from build123d import *

# Parameters (mm, degrees)
SKETCH1_R           = 1.651
BOSS_EXTRUDE1_DEPTH = 3.175
FILLET2_R           = 2.54


with BuildPart() as part:
    # Sketch1 → Boss-Extrude1 (new body)
    with BuildSketch(Plane(origin=(0, 0, 0), x_dir=(1, 0, 0), z_dir=(0, 1, 0))):
        with BuildLine():
            Line((30.48, -63.5), (30.48, 0))
            ThreePointArc((30.48, 0), (0, 30.48), (-30.48, 0))
            Line((-30.48, 0), (-30.48, -63.5))
            Line((-30.48, -63.5), (-1.5875, -63.5))
            Line((-1.5875, -63.5), (-1.5875, -50.8))
            Line((-1.5875, -50.8), (1.5875, -50.8))
            Line((1.5875, -50.8), (1.5875, -63.5))
            Line((1.5875, -63.5), (30.48, -63.5))
        make_face()
        with Locations(Location((-20.447, 0, 0), (0, 0, 270))):
            Circle(SKETCH1_R, mode=Mode.SUBTRACT)
        with BuildLine():
            Line((5.334, -27.813), (-5.334, -27.813))
            Line((-5.334, -27.813), (-5.334, -14.140410638))
            ThreePointArc((-5.334, -14.140410638), (-8.596220885, 12.430114863), (15.113, 0))
            ThreePointArc((15.113, 0), (12.430114863, -8.596220885), (5.334, -14.140410638))
            Line((5.334, -14.140410638), (5.334, -27.813))
        make_face(mode=Mode.SUBTRACT)
        with Locations(Location((20.447, 0, 0), (0, 0, 270))):
            Circle(SKETCH1_R, mode=Mode.SUBTRACT)
    extrude(amount=BOSS_EXTRUDE1_DEPTH)

    # Fillet2
    fillet2_edges = [part.edges().sort_by_distance(p)[0] for p in [
        (-5.334, 1.5875, 14.140410638),
        (-5.334, 1.5875, 27.813),
        (5.334, 1.5875, 27.813),
        (5.334, 1.5875, 14.140410638),
    ]]
    fillet(fillet2_edges, radius=FILLET2_R)


solid = part.part
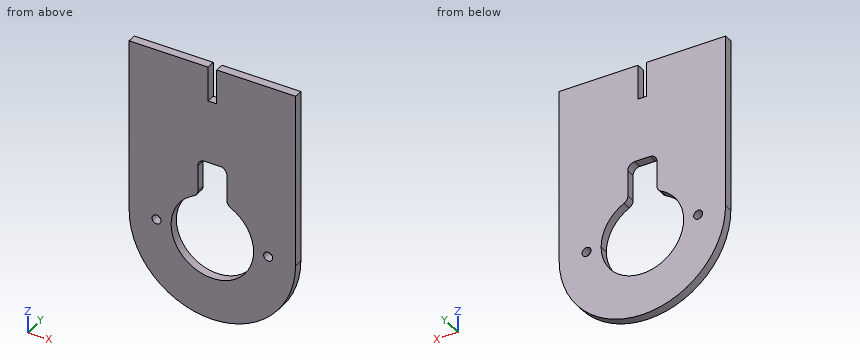
The model under review builds one solid part; all positions refer to its coordinate system, in mm. Round coordinates to 2 decimals unless told otherwise and drop trailing zeros. Loops run counter-clockwise (first coordinate to the right, second up) from the corner with the lowest first, then second, coordinate; pieces in that order, holes last. Notation, with made-up numbers: (89.25, 52) -> (144.25, 52) arc R31 ccw to (144.25, 85) -> close; hole circle Ø7 at (5, 42). An arc over 180 degrees is marked (long way). Return JSON: item names as keys, results as strings.
(1) Add section C-C on y = 1.1. Write out the cut boundary in (x, z).
Solved:
{"outline": "(-30.48, 0) arc R30.48 ccw to (30.48, 0) -> (30.48, 63.5) -> (1.59, 63.5) -> (1.59, 50.8) -> (-1.59, 50.8) -> (-1.59, 63.5) -> (-30.48, 63.5) -> close; hole circle Ø3.3 at (-20.45, 0); hole (-6.74, 13.53) arc R15.11 ccw (long way) to (6.74, 13.53) arc R2.54 cw to (5.33, 15.8) -> (5.33, 25.27) arc R2.54 ccw to (2.79, 27.81) -> (-2.79, 27.81) arc R2.54 ccw to (-5.33, 25.27) -> (-5.33, 15.8) arc R2.54 cw to start; hole circle Ø3.3 at (20.45, 0)"}
(2) Add section A-A on x = 0. Write out the cut boundary in (y, z) (3 decimals), plus the area to 3 significant figures.
Solved:
{"outline": "(0, -30.48) -> (3.175, -30.48) -> (3.175, -15.113) -> (0, -15.113) -> close; (0, 27.813) -> (3.175, 27.813) -> (3.175, 50.8) -> (0, 50.8) -> close", "area": "122 mm2"}
(3) For pin 1 (5.5 mm diameter, centred on x = 20.447, z = 0, fed in from -Y); pin 2 (1 mm diameter, centred on x = 0.5, y = 2, fed in from -Z); pin 3 (2 mm diameter, centred on x = -20.447, z = 0, fed in from +Y), all flat-tipped, find the tip position at first contact; note any pin that passes through.
Solved:
{"pin 1": "y = 0", "pin 2": "z = -30.48", "pin 3": "through"}
(4) Add section B-B on z = 22.5. Write out the cut boundary in (x, y) (3 decimals).
Solved:
{"outline": "(-30.48, 0) -> (-5.334, 0) -> (-5.334, 3.175) -> (-30.48, 3.175) -> close; (5.334, 0) -> (30.48, 0) -> (30.48, 3.175) -> (5.334, 3.175) -> close"}
(5) For line 1 (X direction, y = 0.5, z = 23.5); line 2 (Z direction, x = 0, y = 2.5); line 3 (X direction, y = 3, z = 8.5), list the stretches that pass through material, from the lowest coordinate up.
Solved:
{"line 1": "-30.48 to -5.33, 5.33 to 30.48", "line 2": "-30.48 to -15.11, 27.81 to 50.8", "line 3": "-30.48 to -12.5, 12.5 to 30.48"}
